Read the model definition and answer for the solid it produces. Units are mm, in the model's axes. Face numbers are marked on the shaded views. A direction names the side the tool comes from. Give positions to 0.01 mm unless a question says otherwise; leave off trailing zeros. Loops run counter-clockwise (first coordinate to the right, second up) from the corner with the lowest first, then second, coordinate; pieces in that order, holes last. Notation, with made-up numbers: (-16, -2.5) - (-10, -2.5) arc R23 ccw to (-10, 7.5) - close; hole circle Ø8 at (46, 47). An arc over 180 degrees is marked (long way). Write item = value, one per line.
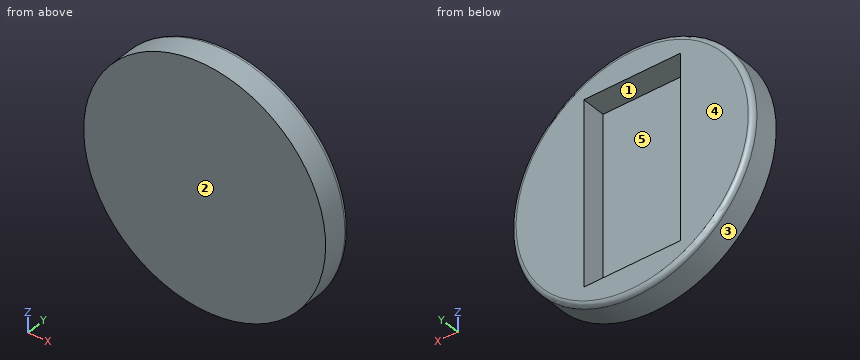
```python
from build123d import *

# Parameters (mm, degrees)
SKETCH1_R           = 25
BOSS_EXTRUDE1_DEPTH = 6
SKETCH2_W           = 20
SKETCH2_H           = 38
CUT_EXTRUDE1_DEPTH  = 5
FILLET1_R           = 1


with BuildPart() as part:
    # Sketch1 → Boss-Extrude1 (new body)
    with BuildSketch(Plane(origin=(0, 0, 0), x_dir=(1, 0, 0), z_dir=(0, 1, 0))):
        with Locations(Location((0, 0, 0), (0, 0, 270))):
            Circle(SKETCH1_R)
    extrude(amount=BOSS_EXTRUDE1_DEPTH)

    # Sketch2 → Cut-Extrude1 (cut)
    with BuildSketch(Plane(origin=(0, 6, 0), x_dir=(1, 0, 0), z_dir=(0, 1, 0))):
        Rectangle(SKETCH2_W, SKETCH2_H)
    extrude(amount=-CUT_EXTRUDE1_DEPTH, mode=Mode.SUBTRACT)

    # Fillet1
    fillet1_edges = [part.edges().sort_by_distance(p)[0] for p in [
        (0, 6, -25),
    ]]
    fillet(fillet1_edges, radius=FILLET1_R)


solid = part.part
```
1) Find the intervals of material crossed by probe 1 along Y at (x, z) = (-5, -10.5); probe 2 along X at (y, z) = (3.35, -7.5); probe 3 along X at (y, z) = (1.9, -1.5), in increasing order.
Output:
probe_1 = 0 to 1
probe_2 = -23.85 to -10, 10 to 23.85
probe_3 = -24.95 to -10, 10 to 24.95
2) A cutting plane is placed at B-B on y = 3.05. Determine the outline of the cut face in (x, z), then the cut area to 3 significant figures.
Output:
outline = circle Ø50 at (0, 0); hole (-10, -19) - (10, -19) - (10, 19) - (-10, 19) - close
area = 1,200 mm²
3) A cutting plane is placed at C-C on z = 0. Determine the outline of the cut face in (x, y).
Output:
outline = (-25, 0) - (25, 0) - (25, 5) arc R1 ccw to (24, 6) - (10, 6) - (10, 1) - (-10, 1) - (-10, 6) - (-24, 6) arc R1 ccw to (-25, 5) - close
4) A cutting plane is placed at A-A on x = 0. Determine the outline of the cut face in (y, z), then the cut area to 3 significant figures.
Output:
outline = (0, -25) - (5, -25) arc R1 ccw to (6, -24) - (6, -19) - (1, -19) - (1, 19) - (6, 19) - (6, 24) arc R1 ccw to (5, 25) - (0, 25) - close
area = 110 mm²
5) Each of these flat-tipped pins is pushed along its axis until it touches: P1, Ø1.5, axis at y = 1.5, z = -6, coming from the -X side; P2, Ø10, axis at x = -2, z = 0.5, coming from the +Y side; P3, Ø1, axis at y = 4, z = -14.5, coming from the -X side. Where does it stop, or does it pass through?
Output:
P1 = -24.44
P2 = 1
P3 = -20.71
6) A tool of negligible diameter and unlimited length cuts with its end or side. For the marked faces 1 and 2, from which of +Z, -Z, +X, -X, +Y, -Y can it reach the whole face along a straight path? Write none if from no direction.
Output:
face_1 = +Y
face_2 = +Z, -Z, +X, -X, -Y
7) The mould has two halves that part along X. Classify the marked faces 3, 4 and 5: pulls with the +X half, pulls with the -X half, needs draft (parallel to the pull), parting line crosses it, or undercut.
Output:
face_3 = parting line crosses it
face_4 = needs draft
face_5 = undercut
